from build123d import *

# Parameters (mm, degrees)
BOSS_EXTRUDE1_DEPTH      = 10
BOSS_EXTRUDE1_DEPTH_BACK = 10
SKETCH2_W                = 3.2
SKETCH2_H                = 20
BOSS_EXTRUDE2_DEPTH      = 10
CUT_EXTRUDE1_START       = -5.2
CUT_EXTRUDE1_DEPTH       = 5.2


# Read off the part's stored shape, not the designer's step: Cut-Extrude1
with BuildPart() as part:
    # Sketch1 → Boss-Extrude1 (new, two sides: drawn at the far end of the back side and taken through both)
    with BuildSketch(Plane.XY.offset(-BOSS_EXTRUDE1_DEPTH_BACK)):
        Polygon((-55, 21.875), (55, -5.625), (55, -8.125), (-55, -8.125), align=None)
    extrude(amount=BOSS_EXTRUDE1_DEPTH + BOSS_EXTRUDE1_DEPTH_BACK)

    # Sketch2 → Boss-Extrude2 (add)
    with BuildSketch(Plane(origin=(1.911764706, 7.647058824, 0), x_dir=(0.970142500145332, -0.24253562503633289, 0), z_dir=(0.24253562503633289, 0.970142500145332, 0))):
        Polygon((-53.463304306, 10), (-50.263304306, 10), (-50.263304306, 2.29875108), (-53.463304306, -2.25), align=None)
        Polygon((-44.863304306, 10), (-44.863304306, 7.5), (-34.863304306, 0.465101973), (-34.863304306, 10), align=None)
        with Locations((18.686695694, 0)):
            Rectangle(SKETCH2_W, SKETCH2_H)
    extrude(amount=BOSS_EXTRUDE2_DEPTH)

    # Cut-Extrude1 outline → Cut-Extrude1 (cut)
    with BuildSketch(Plane.XZ.offset(8.125).offset(CUT_EXTRUDE1_START)):
        Polygon((-14.11294757, -4.9), (-22.553719096, -4.9), (-20.992494606, -10), (-15.67417206, -10), align=None)
        Polygon((14.11294757, -4.9), (15.67417206, -10), (20.992494606, -10), (22.553719096, -4.9), align=None)
    extrude(amount=CUT_EXTRUDE1_DEPTH, mode=Mode.SUBTRACT)


solid = part.part
Here's how the part is built. I have some questions about the finished solid (model axes, mm). A direction names the side the tool comes from. Round coordinates to 2 decimals unless told otherwise and drop trailing zeros. Loops run counter-clockwise (first coordinate to the right, second up) from the corner with the lowest first, then second, coordinate; pieces in that order, holes last. Notation, with made-up numbers: M 59,9.25 L 78,9.25 A33 ccw 78,48.25 Z; hole C 74.5,-3.75 d8. An arc over 180 degrees is marked long. Write each question's results on one line, items separated by ' | '. Start each with the question number.
(1) Will these pins go through, and if not, where does the flat tip stop? P1, Ø2.5, axis at x = 17, y = -4.5, coming from the -Z side; P2, Ø5, axis at x = 22.5, z = -7.5, coming from the +Y side; P3, Ø1.5, axis at x = 19.5, z = -7, coming from the -Y side (3 decimals); P4, Ø8, axis at y = 25.5, z = -7, coming from the -X side.
(2) If I drill on probe 1 along X at (y, z) = (25, -1); probe 2 along Y at (x, z) = (4, 0.5) (3 decimals); probe 3 along Y at (x, z) = (-4, -7) (3 decimals), over which ranges is the centre line in solid material (lowest first)? Write a range as from..to.
(3) I want a section at A-A (x = -30.5). Please give me the cut outline in (y, z) (3 decimals), then the cut area to 3 significant figures.
(4) I want a section at D-D (x = 43.5). Please give me the cut outline in (y, z) (3 decimals).
(5) I want a section at B-B (z = 7.5). Please give me the cut outline in (x, y) (3 decimals).
(6) Thinking about a two-plate mould opening in Y: for faces 1 (the flat face through (-11, 4, 10)), 2 (the flat face through (-47.186, 25.003, -0.056)), 3 (the flat face through (-18, -2.925, -7)), which applies, pulls with the +Y half, pulls with the -Y half, needs draft (parallel to the pull), parting line crosses it, or undercut?
(7) On a 3-axis mill with a long thin cutter (end or side, diameter ignored), from which of +Z, -Z, +X, -X, +Y, -Y can I reach the whole of each face in a straight line? I mean faces 4 (the flat face through (-35.63, 22.12, -4.03)), 5 (the flat face through (-14.904, -5.489, -7.486)), 6 (the flat face through (-45.655, 24.621, -6.203)), 7 (the flat face through (-40.416, 23.311, -8.768)). Say none if no direction works.
(8) I want a section at C-C (y = 6). Please give me the cut outline in (x, z), then the cut area to 3 significant figures.
Solved:
1) P1: stops at z = -4.9 | P2: stops at y = 13.2 | P3: stops at y = -2.925 | P4: stops at x = -55
2) probe 1: x = -48.86..-46.5, -30.47..-29.69 | probe 2: y = -8.125..7.125 | probe 3: y = -8.125..9.125
3) outline: M -8.125,-10 L 15.75,-10 L 15.75,10 L -8.125,10 Z; M 21.745,-10 L 26.058,-10 L 26.058,-1.201 L 21.745,-0.465 Z | area: 517 mm²
4) outline: M -8.125,-10 L -2.75,-10 L -2.75,10 L -8.125,10 Z
5) outline: M -55,-8.125 L 55,-8.125 L 55,-5.625 L 21.593,2.727 L 24.018,12.428 L 20.914,13.204 L 18.488,3.503 L -55,21.875 Z
6) face 1: needs draft | face 2: undercut | face 3: pulls with the -Y half
7) face 4: +Z, +Y | face 5: -Y | face 6: +Z, -Z | face 7: +Z, -Z, +Y
8) outline: M -55,-10 L 8.5,-10 L 8.5,10 L -55,10 Z; M 19.11,-10 L 22.41,-10 L 22.41,10 L 19.11,10 Z | area: 1,340 mm²
